Model file for the job. Use its own axes, mm. A direction names the side the tool comes from. Give positions to 0.01 mm unless a question says otherwise; leave off trailing zeros. Write each loop counter-clockwise with the first axis right and the second up, starting at its lowest first coordinate (ties: lowest second). Pieces come first, ordered by that corner, then holes.
```python
from build123d import *

# Parameters (mm, degrees)
F0_W      = 139.8479826748
F0_H      = 140.0080993772
F1_DEPTH  = 19.05
F2_R      = 5.08
F3_R      = 25.5680364158
F4_DEPTH  = 25.4
F5_DEPTH  = 25.4
F6_T      = -7.62
F7_R      = 25.4280545829
F8_DEPTH  = 25.4
F9_DEPTH  = 25.4
F10_R     = 25.4772603169
F11_DEPTH = 25.4
F12_DEPTH = 25.4
F13_R     = 25.5378066053
F14_DEPTH = 25.4
F15_DEPTH = 25.4


with BuildPart() as f1:
    # F0 (on Top) → F1 (new body)
    with BuildSketch(Plane.XY):
        with Locations((7.7169742435, 24.6758498251)):
            Rectangle(F0_W, F0_H)
    extrude(amount=F1_DEPTH)

    # F2
    f2_edges = [f1.edges().sort_by_distance(p)[0] for p in [
        (7.716974, -45.3282, 19.05),
        (7.716974, -45.3282, 0),
        (-62.207017, 94.6799, 9.525),
        (-62.207017, -45.3282, 9.525),
        (-62.207017, 24.67585, 0),
        (-62.207017, 24.67585, 19.05),
        (7.716974, 94.6799, 19.05),
        (7.716974, 94.6799, 0),
        (77.640966, 24.67585, 19.05),
        (77.640966, 24.67585, 0),
        (77.640966, -45.3282, 9.525),
        (77.640966, 94.6799, 9.525),
    ]]
    fillet(f2_edges, radius=F2_R)

    # F3 (on Top) → F4 (join)
    with BuildSketch(Plane.XY):
        with Locations((-58.9822605252, -41.7709499598)):
            Circle(F3_R)
    extrude(amount=F4_DEPTH)

    # F5 (cut): a face of the model
    f5_faces = [f1.faces().sort_by_distance(p)[0] for p in [
        (-58.9822605252, -41.7709499598, 25.4),
    ]]
    extrude(f5_faces, amount=-F5_DEPTH, mode=Mode.SUBTRACT)

    # F6
    f6_openings = [f1.faces().sort_by_distance(p)[0] for p in [
        (-40.784716, -23.810609, 9.525),
    ]]
    offset(amount=F6_T, openings=f6_openings, kind=Kind.INTERSECTION)

    # F7 (on Top) → F8 (join)
    with BuildSketch(Plane.XY):
        with Locations((-60.7334524393, 92.9428115487)):
            Circle(F7_R)
    extrude(amount=F8_DEPTH)

    # F9 (cut): a face of the model
    f9_faces = [f1.faces().sort_by_distance(p)[0] for p in [
        (-60.7334524393, 92.9428115487, 25.4),
    ]]
    extrude(f9_faces, amount=-F9_DEPTH, mode=Mode.SUBTRACT)

    # F10 (on Top) → F11 (join)
    with BuildSketch(Plane.XY):
        with Locations((76.0564357042, -43.5319244862)):
            Circle(F10_R)
    extrude(amount=F11_DEPTH)

    # F12 (cut): a face of the model
    f12_faces = [f1.faces().sort_by_distance(p)[0] for p in [
        (76.0564357042, -43.5319244862, 25.4),
    ]]
    extrude(f12_faces, amount=-F12_DEPTH, mode=Mode.SUBTRACT)

    # F13 (on Top) → F14 (join)
    with BuildSketch(Plane.XY):
        with Locations((75.2917006612, 93.2972580194)):
            Circle(F13_R)
    extrude(amount=F14_DEPTH)

    # F15 (cut): a face of the model
    f15_faces = [f1.faces().sort_by_distance(p)[0] for p in [
        (75.2917006612, 93.2972580194, 25.4),
    ]]
    extrude(f15_faces, amount=-F15_DEPTH, mode=Mode.SUBTRACT)


solid = f1.part
```
1. Pin check, flat tips, straight feed: P1, Ø5, axis at x = 57.5, z = 13, coming from the -Y side; P2, Ø1.5, axis at y = -27, z = 4, coming from the +X side. Stop position of each tip, or through.
Calculated:
P1: stops at y = -29.19
P2: stops at x = 57.34
2. Which spindle directions (+Z, -Z, +X, -X, +Y, -Y) get a long thin tool onto all of the face, cutting with end or side? Do faces 1 (the cylindrical face through (-60.76, 26.27, 1.53)), 2 (the flat face through (7, 26, 7.62)), 3 (the flat face through (7, 87.06, 9)), 4 (the cylindrical face through (76.192, 25.409, 1.528)), 5 (the flat face through (-54.587, 25, 9)). Say none if no direction does.
Calculated:
face 1: -Z, -X, +Y, -Y
face 2: none
face 3: +X, -X
face 4: -Z, +X, +Y, -Y
face 5: +Y, -Y
3. Probe probe 1 along Z at (x, y) = (-31, -5); probe 2 along Y at (x, z) = (-28.5, 10.75); probe 3 along X at (y, z) = (31.5, 11.25). List the from-to ranges inside material, lowest first.
Calculated:
probe 1: z = 0 to 7.62, 11.43 to 19.05
probe 2: y = -45.33 to -37.71, 87.06 to 94.68
probe 3: x = -62.21 to -54.59, 70.02 to 77.64
4. Slice it at C-C, the plane x = -40.5. Write the cut outline in (y, z).
Calculated:
outline: (-24.1, 0) - (77.54, 0) - (77.54, 7.62) - (-24.1, 7.62) - close; (-24.1, 11.43) - (77.54, 11.43) - (77.54, 19.05) - (-24.1, 19.05) - close
5. Pull direction X, two halves, no side cores. Call faces 6 (the cylindrical face through (-40.6, -24, 11.8)), 7 (the cylindrical face through (-60.76, 26.27, 17.52)), 8 (the cylindrical face through (9.2, -43.9, 17.5)): +X half, -X half, draft (parallel to the pull), parting line (faces both ways), or undercut.
Calculated:
face 6: undercut
face 7: -X half
face 8: draft
6. Slice it at A-A, the plane y = 78. Write the cut outline in (x, z).
Calculated:
outline: (-40.16, 0) - (54.84, 0) - (54.84, 7.62) - (-40.16, 7.62) - close; (-40.16, 11.43) - (54.84, 11.43) - (54.84, 19.05) - (-40.16, 19.05) - close
7. Slice it at D-D, the plane y = 7. Write the cut outline in (x, z), and give its area (3 significant figures).
Calculated:
outline: (-62.21, 5.08) arc R5.08 ccw to (-57.13, 0) - (72.56, 0) arc R5.08 ccw to (77.64, 5.08) - (77.64, 13.97) arc R5.08 ccw to (72.56, 19.05) - (-57.13, 19.05) arc R5.08 ccw to (-62.21, 13.97) - close; hole (-54.59, 7.62) - (70.02, 7.62) - (70.02, 11.43) - (-54.59, 11.43) - close
area: 2,170 mm2
8. Slice it at B-B, the plane x = -18.5. Write the cut outline in (y, z), and give its area (3 significant figures).
Calculated:
outline: (-45.33, 5.08) arc R5.08 ccw to (-40.25, 0) - (89.6, 0) arc R5.08 ccw to (94.68, 5.08) - (94.68, 13.97) arc R5.08 ccw to (89.6, 19.05) - (-40.25, 19.05) arc R5.08 ccw to (-45.33, 13.97) - close; hole (-37.71, 7.62) - (87.06, 7.62) - (87.06, 11.43) - (-37.71, 11.43) - close
area: 2,170 mm2
